Could you check a few things on this model? Use its own coordinates, in mm. Face numbers are marked on the shaded views. Coordinates: 2 decimals unless noted, no trailing zeros. Order: outer loops, then holes, each group sorted by start corner. A loop starts at its lowest first (then second) coordinate and runs counter-clockwise, first axis right, second up. Notation, with made-up numbers: (-34.5, 31) -> (-12.5, 31) arc R10 ccw to (-12.5, 38) -> close; hole circle Ø1 at (27.25, 45). An arc over 180 degrees is marked (long way). Put each result on its own line as item: value. Start each with the question number.
Q1. If we section it at A-A (x = 47): Please give me the cut outline in (y, z), and give its area (3 significant figures).
Q2. We'd pull the mould along X, two halves only. Please class the marked faces 1, 2, 3 and 4: +X half, -X half, draft (parallel to the pull), parting line (faces both ways), or undercut.
Q3. If we section it at D-D (x = 0): Please give me the cut outline in (y, z).
Q4. If we section it at C-C (z = 24): Please give me the cut outline in (x, y).
Q5. Will these pins go through, and if not, where does the flat tip stop? pin 1 (10 mm diameter, centred on x = -17.5, y = -13.5, fed in from -Z); pin 2 (12.5 mm diameter, centred on x = -47, z = 26, fed in from -Y); pin 3 (10 mm diameter, centred on y = -11.5, z = 24, fed in from +X); pin 4 (12 mm diameter, centred on y = -17, z = -54, fed in from +X).
Q6. If we section it at B-B (z = -65): Please give me the cut outline in (x, y).
Q7. Please list where these lines run through material, in increasing order: line 1 along Z through (x, y) = (0, -11.5); line 2 along Z through (x, y) = (-47, -6.5); line 3 along Z through (x, y) = (-3.5, -14.5).
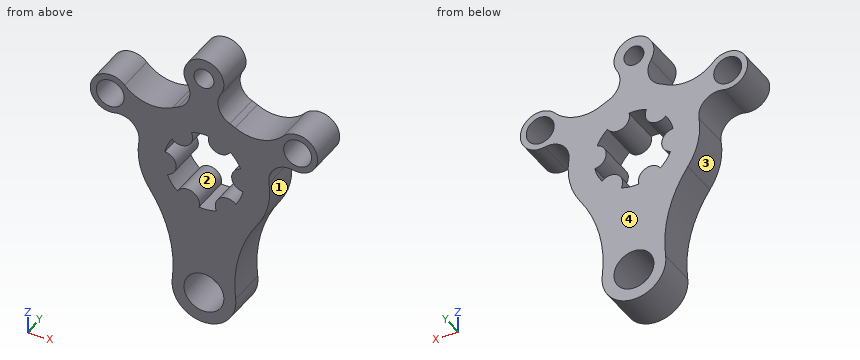
Autodesk Fusion 360 part; units mm, degrees
sketch "Sketch1" plane through (0, 0, 0) normal (0, 1, 0) x (1, 0, 0)
  circle A0 centre (0, 65) radius 10
  circle A1 centre (0, -50) radius 5
  circle A2 centre (-47, -26) radius 7
  arc A3 (-27.0298, 18.9312) -> (-15.8903, 63.1292) centre (-79.4513, 55.6462) ccw
  arc A4 (-44.752, -16.2559) -> (-32.6194, -4.9975) centre (-42.5041, -6.5119) ccw
  arc A5 (-15.6968, -29.0277) -> (-39.7367, -32.8734) centre (-25.21, -46.6203) ccw
  arc A6 (-8.5079, -44.745) -> (-13.0587, -30.3063) centre (-17.0159, -39.49) ccw
  arc A7 (-15.6968, -29.0277) -> (-13.0587, -30.3063) centre (0, 0) ccw
  arc A8 (-27.0298, 18.9312) -> (-32.6194, -4.9975) centre (0, 0) ccw
  arc A9 (15.8903, 63.1292) -> (-15.8903, 63.1292) centre (0, 65) ccw
  arc A10 (-44.752, -16.2559) -> (-39.7367, -32.8734) centre (-47, -26) ccw
  arc A11 (-8.5079, -44.745) -> (8.5079, -44.745) centre (0, -50) ccw
  arc A12 (15.8903, 63.1292) -> (27.0298, 18.9312) centre (79.4513, 55.6462) ccw
  arc A13 (32.6194, -4.9975) -> (27.0298, 18.9312) centre (0, 0) ccw
  arc A14 (32.6194, -4.9975) -> (44.752, -16.2559) centre (42.5041, -6.5119) ccw
  arc A15 (39.7367, -32.8734) -> (44.752, -16.2559) centre (47, -26) ccw
  circle A16 centre (47, -26) radius 7
  arc A17 (39.7367, -32.8734) -> (15.6968, -29.0277) centre (25.21, -46.6203) ccw
  arc A18 (13.0587, -30.3063) -> (15.6968, -29.0277) centre (0, 0) ccw
  arc A19 (13.0587, -30.3063) -> (8.5079, -44.745) centre (17.0159, -39.49) ccw
  arc A20 (-13.27, 14.9635) -> (-2.4581, 19.8484) centre (-8.2346, 18.2261) ccw
  arc A21 (-19.5938, -4.0104) -> (-18.4182, 7.7954) centre (-19.9016, 1.9817) ccw
  arc A22 (-6.3238, -18.9739) -> (-15.9602, -12.0529) centre (-11.667, -16.2444) ccw
  arc A23 (13.27, -14.9635) -> (2.4581, -19.8484) centre (8.2346, -18.2261) ccw
  arc A24 (19.5938, 4.0104) -> (18.4182, -7.7954) centre (19.9016, -1.9817) ccw
  arc A25 (6.3238, 18.9739) -> (15.9602, 12.0529) centre (11.667, 16.2444) ccw
  arc A26 (6.3238, 18.9739) -> (-2.4581, 19.8484) centre (0, 0) ccw
  arc A27 (19.5938, 4.0104) -> (15.9602, 12.0529) centre (0, 0) ccw
  arc A28 (13.27, -14.9635) -> (18.4182, -7.7954) centre (0, 0) ccw
  arc A29 (-6.3238, -18.9739) -> (2.4581, -19.8484) centre (0, 0) ccw
  arc A30 (-13.27, 14.9635) -> (-18.4182, 7.7954) centre (0, 0) ccw
  arc A31 (-19.5938, -4.0104) -> (-15.9602, -12.0529) centre (0, 0) ccw
  dimension "d1" = 66
  dimension "d2" = 40
  dimension "d3" = 32
  dimension "d4" = 20
  dimension "d5" = 65
  dimension "d6" = 20
  dimension "d7" = 10
  dimension "d8" = 14
  dimension "d9" = 20
  dimension "d10" = 26
  dimension "d11" = 24
  dimension "d12" = 47
  dimension "d13" = 128
  dimension "d14" = 20
  dimension "d15" = 40
  dimension "d16" = 20
  dimension "d17" = 12
  dimension "d19" = 360
extrude "Extrude1" add sketch "Sketch1" against normal blind 20
The answers:
1. outline: (-20, 16) -> (0, 16) -> (0, 19) -> (-20, 19) -> close; (-20, 33) -> (0, 33) -> (0, 36) -> (-20, 36) -> close
1. area: 120 mm^2
2. face 1: +X half
2. face 2: undercut
2. face 3: -X half
2. face 4: draft
3. outline: (-20, -81) -> (0, -81) -> (0, -75) -> (-20, -75) -> close; (-20, -55) -> (0, -55) -> (0, -20) -> (-20, -20) -> close; (-20, 20) -> (0, 20) -> (0, 45) -> (-20, 45) -> close; (-20, 55) -> (0, 55) -> (0, 60) -> (-20, 60) -> close
4. outline: (-56.8, -20) -> (-53.71, -20) -> (-53.71, 0) -> (-56.8, 0) -> close; (-40.29, -20) -> (40.29, -20) -> (40.29, 0) -> (-40.29, 0) -> close; (53.71, -20) -> (56.8, -20) -> (56.8, 0) -> (53.71, 0) -> close
5. pin 1: z = -74.99
5. pin 2: through
5. pin 3: x = 57
5. pin 4: x = 15.91
6. outline: (-16, -20) -> (-10, -20) -> (-10, 0) -> (-16, 0) -> close; (10, -20) -> (16, -20) -> (16, 0) -> (10, 0) -> close
7. line 1: -81 to -75, -55 to -20, 20 to 45, 55 to 60
7. line 2: 16 to 19, 33 to 36
7. line 3: -80.61 to -74.37, -55.63 to -14.54, 19.69 to 46.43, 53.57 to 59.37
